from build123d import *

# Parameters (mm, degrees)
SKETCH_1_W          = 225
SKETCH_1_H          = 155
EXTRUDE_1_DEPTH     = 80
FILLET_1_R          = 3
SHELL_1_T           = -2
SKETCH_2_R          = 3.5
SKETCH_2_R_2        = 1.25
EXTRUDE_2_DEPTH     = 5
SKETCH_4_W          = 28.5
SKETCH_4_H          = 39.5
CUT_EXTRUDE_3_DEPTH = 3
FILLET_2_R          = 2
SKETCH_5_R          = 10
CUT_EXTRUDE_4_DEPTH = 3
SKETCH_6_R          = 3.75
CUT_EXTRUDE_5_DEPTH = 3
CUT_EXTRUDE_6_DEPTH = 3
CUT_EXTRUDE_7_DEPTH = 1
SKETCH_9_R          = 3.5
EXTRUDE_4_DEPTH     = 3
SKETCH_10_R         = 1.25
CUT_EXTRUDE_8_DEPTH = 5
CUT_EXTRUDE_START   = -2
SKETCH_11_R         = 1.25
CUT_EXTRUDE_9_DEPTH = 2


with BuildPart() as part:
    # 草图1 → 凸台-拉伸1 (new body)
    with BuildSketch(Plane.XY):
        with Locations((112.5, -77.5)):
            Rectangle(SKETCH_1_W, SKETCH_1_H)
    extrude(amount=EXTRUDE_1_DEPTH)

    # 圆角1
    fillet_1_edges = [part.edges().sort_by_distance(p)[0] for p in [
        (0, 0, 40),
        (225, 0, 40),
        (225, -155, 40),
        (0, -155, 40),
    ]]
    fillet(fillet_1_edges, radius=FILLET_1_R)

    # 抽壳1
    shell_1_openings = [part.faces().sort_by_distance(p)[0] for p in [
        (112.5, -77.5, 80),
    ]]
    offset(amount=SHELL_1_T, openings=shell_1_openings, kind=Kind.INTERSECTION)

    # 草图2 → 凸台-拉伸2 (add)
    # profile 1 of 4: a face of its own
    with BuildSketch(Plane.XY.offset(2)):
        with Locations((217, -20)):
            Circle(SKETCH_2_R)
        with Locations((217, -20)):
            Circle(SKETCH_2_R_2, mode=Mode.SUBTRACT)
    # profile 2 of 4: a face of its own
    with BuildSketch(Plane.XY.offset(2)):
        with Locations((152, -20)):
            Circle(SKETCH_2_R)
        with Locations((152, -20)):
            Circle(SKETCH_2_R_2, mode=Mode.SUBTRACT)
    # profile 3 of 4: a face of its own
    with BuildSketch(Plane.XY.offset(2)):
        with Locations((152, -135)):
            Circle(SKETCH_2_R)
        with Locations((152, -135)):
            Circle(SKETCH_2_R_2, mode=Mode.SUBTRACT)
    # profile 4 of 4: a face of its own
    with BuildSketch(Plane.XY.offset(2)):
        with Locations((217, -135)):
            Circle(SKETCH_2_R)
        with Locations((217, -135)):
            Circle(SKETCH_2_R_2, mode=Mode.SUBTRACT)
    extrude(amount=EXTRUDE_2_DEPTH)

    # 草图4 → 切除-拉伸3 (cut)
    with BuildSketch(Plane(origin=(225, 0, 0), x_dir=(0, 0, -1), z_dir=(1, 0, 0))):
        with Locations((-54.25, -42.75)):
            Rectangle(SKETCH_4_W, SKETCH_4_H)
    extrude(amount=-CUT_EXTRUDE_3_DEPTH, mode=Mode.SUBTRACT)

    # 圆角2
    fillet_2_edges = [part.edges().sort_by_distance(p)[0] for p in [
        (224, -62.5, 68.5),
        (224, -23, 68.5),
        (224, -23, 40),
        (224, -62.5, 40),
    ]]
    fillet(fillet_2_edges, radius=FILLET_2_R)

    # 草图5 → 切除-拉伸4 (cut)
    with BuildSketch(Plane.ZY):
        with Locations((29, -77.5)):
            Circle(SKETCH_5_R)
    extrude(amount=-CUT_EXTRUDE_4_DEPTH, mode=Mode.SUBTRACT)

    # 草图6 → 切除-拉伸5 (cut)
    with BuildSketch(Plane(origin=(225, 0, 0), x_dir=(0, 0, -1), z_dir=(1, 0, 0))):
        with Locations(Location((-54.25, -107.25, 0), (0, 0, 90))):
            Circle(SKETCH_6_R)
    extrude(amount=-CUT_EXTRUDE_5_DEPTH, mode=Mode.SUBTRACT)

    # 草图7 → 切除-拉伸6 (cut)
    with BuildSketch(Plane.ZY):
        with BuildLine():
            Line((31, -133), (31, -137))
            ThreePointArc((31, -137), (29, -139), (27, -137))
            Line((27, -137), (27, -133))
            ThreePointArc((27, -133), (29, -131), (31, -133))
        make_face()
    extrude(amount=-CUT_EXTRUDE_6_DEPTH, mode=Mode.SUBTRACT)

    # 草图8 → 切除-拉伸7 (cut)
    with BuildSketch(Plane.XY.offset(80)):
        with BuildLine():
            Line((3, -154), (222, -154))
            ThreePointArc((222, -154), (223.414213562, -153.414213562), (224, -152))
            Line((224, -152), (224, -3))
            ThreePointArc((224, -3), (223.414213562, -1.585786438), (222, -1))
            Line((222, -1), (3, -1))
            ThreePointArc((3, -1), (1.585786438, -1.585786438), (1, -3))
            Line((1, -3), (1, -152))
            ThreePointArc((1, -152), (1.585786438, -153.414213562), (3, -154))
        make_face()
        with BuildLine():
            Line((3, -153), (222, -153))
            ThreePointArc((222, -153), (222.707106781, -152.707106781), (223, -152))
            Line((223, -152), (223, -3))
            ThreePointArc((223, -3), (222.707106781, -2.292893219), (222, -2))
            Line((222, -2), (3, -2))
            ThreePointArc((3, -2), (2.292893219, -2.292893219), (2, -3))
            Line((2, -3), (2, -152))
            ThreePointArc((2, -152), (2.292893219, -152.707106781), (3, -153))
        make_face(mode=Mode.SUBTRACT)
    extrude(amount=-CUT_EXTRUDE_7_DEPTH, mode=Mode.SUBTRACT)

    # 草图9 → 凸台-拉伸4 (add)
    with BuildSketch(Plane.XY.offset(2)):
        with Locations((15, -10)):
            Circle(SKETCH_9_R)
        with Locations((210, -10)):
            Circle(SKETCH_9_R)
        with Locations((210, -145)):
            Circle(SKETCH_9_R)
        with Locations((15, -145)):
            Circle(SKETCH_9_R)
    extrude(amount=EXTRUDE_4_DEPTH)

    # 草图10 → 切除-拉伸8 (cut)
    with BuildSketch(Plane.XY.offset(5)):
        with Locations((15, -10)):
            Circle(SKETCH_10_R)
        with Locations((210, -10)):
            Circle(SKETCH_10_R)
        with Locations((210, -145)):
            Circle(SKETCH_10_R)
        with Locations((15, -145)):
            Circle(SKETCH_10_R)
    extrude(amount=-CUT_EXTRUDE_8_DEPTH, mode=Mode.SUBTRACT)

    # 草图11 → 切除-拉伸9 (cut)
    with BuildSketch(Plane.XY.offset(2).offset(CUT_EXTRUDE_START)):
        with Locations((217, -20)):
            Circle(SKETCH_11_R)
        with Locations((152, -20)):
            Circle(SKETCH_11_R)
        with Locations((217, -135)):
            Circle(SKETCH_11_R)
        with Locations((152, -135)):
            Circle(SKETCH_11_R)
    extrude(amount=CUT_EXTRUDE_9_DEPTH, mode=Mode.SUBTRACT)


solid = part.part
Check sheet for the modelled part. Datum: model origin and axes. Units: mm. A direction names the side the tool comes from. Round coordinates to 2 decimals unless told otherwise and drop trailing zeros. Order: outer loops, then holes, each group sorted by start corner. A loop starts at its lowest first (then second) coordinate and runs counter-clockwise, first axis right, second up.
(1) Cross-section at D-D, the plane y = -29.5. Enter the section's corners in (x, z), and give its area (3 significant figures).
(2) Cross-section at A-A, the plane y = -107.25. Enter the section's corners in (x, z), and give its area (3 significant figures).
(3) Go/stop test with flat-tipped pins: P1, Ø3.5, axis at x = 208.5, y = -144, coming from the +Z side; P2, Ø3.5, axis at x = 218, y = -20, coming from the +Z side; P3, Ø4, axis at y = -51.5, z = 66, coming from the +X side. Record where each tip stops, or that it passes through.
(4) Scan lines: probe 1 along Y at (x, z) = (15, 1.85); probe 2 along X at (y, z) = (-145, 1.85); probe 3 along Y at (x, z) = (152, 2.75). Record each from-to range of solid material in increasing order.
(5) Access from +Z, -Z, +X, -X, +Y, -Y to the whole of each face (thin tool, end or side, straight path). Record for faces 1 (the flat face through (111, -76, 2)), 2 (the cylindrical face through (0.99, -69.07, 34.38)), 3 (the flat face through (111, -155, 39)).
(6) Cross-section at B-B, the plane z = 54.25. Enter the section's corners in (x, y), and give its area (3 significant figures).
(7) Draft check along X on faces 4 (the cylindrical face through (224.014, -105.52, 50.923)), 5 (the flat face through (0, -78.5, 39.4)), 6 (the cylindrical face through (155.34, -18.95, 4.46)). Enter one of: pulls with the +X half, pulls with the -X half, needs draft (parallel to the pull), parting line crosses it, or undercut.
(8) Cross-section at C-C, the plane x = 73. Enter the section's corners in (y, z), and give its area (3 significant figures).
Check sheet entries:
1. outline: (0, 0) - (225, 0) - (225, 40) - (223, 40) - (223, 2) - (2, 2) - (2, 79) - (1, 79) - (1, 80) - (0, 80) - close; (223, 68.5) - (225, 68.5) - (225, 80) - (224, 80) - (224, 79) - (223, 79) - close
1. area: 703 mm2
2. outline: (0, 0) - (225, 0) - (225, 50.5) - (223, 50.5) - (223, 2) - (2, 2) - (2, 79) - (1, 79) - (1, 80) - (0, 80) - close; (223, 58) - (225, 58) - (225, 80) - (224, 80) - (224, 79) - (223, 79) - close
2. area: 745 mm2
3. P1: stops at z = 5
3. P2: stops at z = 7
3. P3: stops at x = 2
4. probe 1: y = -155 to -146.25, -143.75 to -11.25, -8.75 to 0
4. probe 2: x = 0 to 13.75, 16.25 to 208.75, 211.25 to 225
4. probe 3: y = -155 to -153, -138.5 to -136.25, -133.75 to -131.5, -23.5 to -21.25, -18.75 to -16.5, -2 to 0
5. face 1: +Z
5. face 2: -X
5. face 3: +Z, -Z, +X, -X, -Y
6. outline: (0, -152) arc R3 ccw to (3, -155) - (222, -155) arc R3 ccw to (225, -152) - (225, -111) - (223, -111) - (223, -152) arc R1 cw to (222, -153) - (3, -153) arc R1 cw to (2, -152) - (2, -3) arc R1 cw to (3, -2) - (222, -2) arc R1 cw to (223, -3) - (223, -23) - (225, -23) - (225, -3) arc R3 ccw to (222, 0) - (3, 0) arc R3 ccw to (0, -3) - close; (223, -103.5) - (225, -103.5) - (225, -62.5) - (223, -62.5) - close
6. area: 1,400 mm2
7. face 4: needs draft
7. face 5: pulls with the -X half
7. face 6: undercut
8. outline: (-155, 0) - (0, 0) - (0, 80) - (-1, 80) - (-1, 79) - (-2, 79) - (-2, 2) - (-153, 2) - (-153, 79) - (-154, 79) - (-154, 80) - (-155, 80) - close
8. area: 620 mm2
